Source: CAD feature listing. Evaluate the final solid. Frame: model axes, mm. A direction names the side the tool comes from. Coordinates: 2 decimals unless noted, no trailing zeros. Order: outer loops, then holes, each group sorted by start corner. A loop starts at its lowest first (then second) coordinate and runs counter-clockwise, first axis right, second up.
Item 1: Section A-A on y = 7.5. State how many separate pieces and enclosed holes the cut face has, then the cut area to 3 significant figures.
Item 2: Reachability of faces 4 (the flat face through (-11, 7, -3)), 5 (the flat face through (0, 7, 0)), 6 (the flat face through (5, 0, -2)) from +Z, -Z, +X, -X, +Y, -Y: full face, straight path, thin tool, end or side. Return the list, or none.
Item 3: Section B-B on x = 14. Return the cut outline in (y, z).
Item 4: Mould query, pull axis X, two halves, no side actions, for faces 1 (the flat face through (17, 7, -3)), 2 (the flat face through (-20, 7, -1)), 3 (the cylindrical face through (-12.851, 5.292, -1.479)). Classes: released by +X, released by -X, zero draft, split by the parting line, or undercut.
Item 5: Ray query, line 1 (Y direction, x = 14, z = -1.6); line 2 (Z direction, x = 18.5, y = 3.5); line 3 (Y direction, x = -7.5, z = -0.25). Return the intervals inside material, ascending.
Item 6: Section C-C on z = -5. Return the cut outline in (x, y).
Item 7: Contact query for flat-ended pins moving along their axis: P1, Ø4.5, axis at x = 14, y = 7.5, coming from the +Z side; P2, Ø6, axis at x = 13, y = 6, coming from the -Z side; P3, Ø4, axis at y = -6, z = -7.5, coming from the +X side; P4, Ø3, axis at x = -8, z = -2, coming from the -Y side. Output: stop coordinate, or through.
from build123d import *
from build123d.topology import SkipClean

# Parameters (mm, degrees)
BOSS_EXTRUDE1_DEPTH    = 15
FILLET1_R              = 3.175
SKETCH2_R              = 4.7625
BOSS_EXTRUDE2_DEPTH    = 33
FILLET2_R              = 1
F_10_CLEARANCE_HOLE1_D = 4.9784


with BuildPart() as part:
    # Sketch1 → Boss-Extrude1 (new body)
    with BuildSketch(Plane(origin=(0, 0, 0), x_dir=(1, 0, 0), z_dir=(0, 1, 0))):
        with BuildLine():
            Line((-20, 3), (-4.322199, 3))
            ThreePointArc((-4.322199, 3), (0, 9.7625), (4.322199, 3))
            Line((4.322199, 3), (20, 3))
            Line((20, 3), (20, 0))
            Line((20, 0), (-20, 0))
            Line((-20, 0), (-20, 3))
        make_face()
    extrude(amount=BOSS_EXTRUDE1_DEPTH)

    # Fillet1
    fillet1_edges = [part.edges().sort_by_distance(p)[0] for p in [
        (-4.322199, 7.5, -3),
        (4.322199, 7.5, -3),
    ]]
    fillet(fillet1_edges, radius=FILLET1_R)

    # Sketch2 → Boss-Extrude2 (add)
    with SkipClean():  # keep this step's faces unmerged: merging them makes the solid invalid here
        with BuildSketch(Plane.XZ):
            with Locations(Location((0, -5, 0), (0, 0, 270))):  # turned: the seam where the file's is
                Circle(SKETCH2_R)
        extrude(amount=BOSS_EXTRUDE2_DEPTH)

    # Fillet2
    fillet2_edges = [part.edges().sort_by_distance(p)[0] for p in [
        (0, -33, -0.2375),
    ]]
    fillet(fillet2_edges, radius=FILLET2_R)

    # #10 Clearance Hole1 (through all)
    with Locations(Plane(origin=(0, 0, -3), x_dir=(-1, 0, 0), z_dir=(0, 0, -1))):
        with Locations((14, 7.5), (-14, 7.5)):
            Hole(F_10_CLEARANCE_HOLE1_D / 2)


solid = part.part
Answer list:
1. separate pieces: 3
1. enclosed holes: 0
1. area: 149 mm2
2. face 4: -Z, -X, +Y, -Y
2. face 5: +Z, +X, -X, +Y, -Y
2. face 6: +Z, -Y
3. outline: (0, -3) - (5.01, -3) - (5.01, 0) - (0, 0) - close; (9.99, -3) - (15, -3) - (15, 0) - (9.99, 0) - close
4. face 1: zero draft
4. face 2: released by -X
4. face 3: undercut
5. line 1: y = 0 to 5.01, 9.99 to 15
5. line 2: z = -3 to 0
5. line 3: y = 0 to 15
6. outline: (-4.9, 0) - (-4.76, 0) - (-4.76, -32) arc R1 ccw to (-3.76, -33) - (3.76, -33) arc R1 ccw to (4.76, -32) - (4.76, 0) - (4.9, 0) - (4.9, 15) - (-4.9, 15) - close
7. P1: passes through
7. P2: stops at z = -3
7. P3: stops at x = 4.74
7. P4: stops at y = 0
